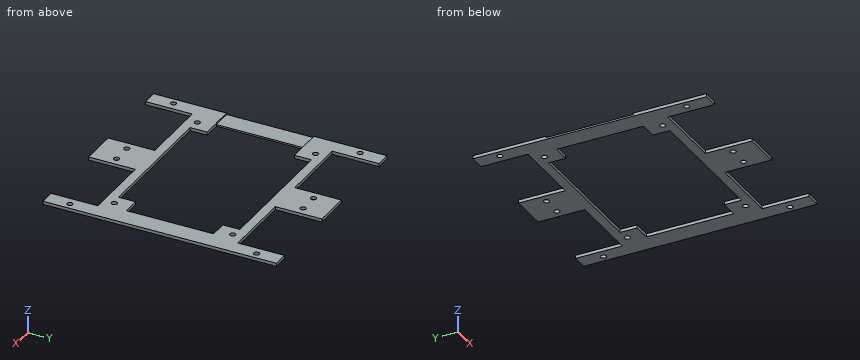
from build123d import *

# Parameters (mm, degrees)
SKETCH2_W           = 680
SKETCH2_H           = 750
BOSS_EXTRUDE1_DEPTH = 10
SKETCH3_W           = 230
SKETCH3_H           = 150
CUT_EXTRUDE1_DEPTH  = 507.285492583
SKETCH4_R           = 9
CUT_EXTRUDE4_DEPTH  = 507.285492583
SKETCH6_W           = 440
SKETCH6_H           = 280
SKETCH6_H_2         = 55
SKETCH6_W_2         = 56.5
CUT_EXTRUDE6_DEPTH  = 507.285492583
SKETCH7_W           = 63.5
SKETCH7_H           = 280.49751631
CUT_EXTRUDE7_DEPTH  = 4.6


with BuildPart() as part:
    # Sketch2 → Boss-Extrude1 (new body)
    with BuildSketch(Plane.XY):
        Rectangle(SKETCH2_W, SKETCH2_H)
    extrude(amount=BOSS_EXTRUDE1_DEPTH)

    # Sketch3 → Cut-Extrude1 (cut, through all)
    with BuildSketch(Plane.XY.offset(10)):
        with Locations((-175, 300)):
            Rectangle(SKETCH3_W, SKETCH3_H)
        with Locations((175, 300)):
            Rectangle(SKETCH3_W, SKETCH3_H)
        with Locations((175, -300)):
            Rectangle(SKETCH3_W, SKETCH3_H)
        with Locations((-175, -300)):
            Rectangle(SKETCH3_W, SKETCH3_H)
    extrude(amount=-CUT_EXTRUDE1_DEPTH, mode=Mode.SUBTRACT)

    # Sketch4 → Cut-Extrude4 (cut, through all)
    with BuildSketch(Plane.XY.offset(10)):
        with Locations((-318, 300)):
            Circle(SKETCH4_R)
        with Locations((-32, 300)):
            Circle(SKETCH4_R)
        with Locations((-255, 190)):
            Circle(SKETCH4_R)
        with Locations(Location((318, 300, 0), (0, 0, 180))):
            Circle(SKETCH4_R)
        with Locations(Location((255, 190, 0), (0, 0, 180))):
            Circle(SKETCH4_R)
        with Locations(Location((32, 300, 0), (0, 0, 180))):
            Circle(SKETCH4_R)
        with Locations((318, -300)):
            Circle(SKETCH4_R)
        with Locations((255, -190)):
            Circle(SKETCH4_R)
        with Locations((32, -300)):
            Circle(SKETCH4_R)
        with Locations(Location((-255, -190, 0), (0, 0, 180))):
            Circle(SKETCH4_R)
        with Locations(Location((-32, -300, 0), (0, 0, 180))):
            Circle(SKETCH4_R)
        with Locations(Location((-318, -300, 0), (0, 0, 180))):
            Circle(SKETCH4_R)
    extrude(amount=-CUT_EXTRUDE4_DEPTH, mode=Mode.SUBTRACT)

    # Sketch6 → Cut-Extrude6 (cut, through all)
    with BuildSketch(Plane.XY.offset(10)):
        Rectangle(SKETCH6_W, SKETCH6_H)
        with Locations((0, 167.5)):
            Rectangle(SKETCH6_W, SKETCH6_H_2)
        with Locations((0, -167.5)):
            Rectangle(SKETCH6_W, SKETCH6_H_2)
        with Locations((248.25, 0)):
            Rectangle(SKETCH6_W_2, SKETCH6_H)
        with Locations((-248.25, 0)):
            Rectangle(SKETCH6_W_2, SKETCH6_H)
    extrude(amount=-CUT_EXTRUDE6_DEPTH, mode=Mode.SUBTRACT)

    # Sketch7 → Cut-Extrude7 (cut)
    with BuildSketch(Plane.XY.offset(10)):
        with Locations((-308.25, -0.248758155)):
            Rectangle(SKETCH7_W, SKETCH7_H)
    extrude(amount=-CUT_EXTRUDE7_DEPTH, mode=Mode.SUBTRACT)


solid = part.part
Input: part model. Units: mm. Frame: model coordinates. Give positions to 0.01 mm unless a question says otherwise; leave off trailing zeros. Loops run counter-clockwise (first coordinate to the right, second up) from the corner with the lowest first, then second, coordinate; pieces in that order, holes last. Notation, with made-up numbers: M 42,-34.5 L 82,-34.5 A18 cw 82,-2.5 Z; hole C 24,-35 d7. An arc over 180 degrees is marked long. Use one line per item in the form item = value.
1. Section query D-D, the plane y = 300. Return the cut outline in (x, z), and give its area (3 significant figures).
Numbers:
outline = M -340,0 L -327,0 L -327,10 L -340,10 Z; M -309,0 L -290,0 L -290,10 L -309,10 Z; M -60,0 L -41,0 L -41,10 L -60,10 Z; M -23,0 L 23,0 L 23,10 L -23,10 Z; M 41,0 L 60,0 L 60,10 L 41,10 Z; M 290,0 L 309,0 L 309,10 L 290,10 Z; M 327,0 L 340,0 L 340,10 L 327,10 Z
area = 1,480 mm²
2. Section query B-B, the plane y = -110. Return the cut outline in (x, z).
Numbers:
outline = M -340,0 L -276.5,0 L -276.5,5.4 L -340,5.4 Z; M 276.5,0 L 340,0 L 340,10 L 276.5,10 Z
3. First-contact query: pin 1 (3 mm diameter, centred on x = 233.5, z = 1.5, fed in from -Y); pin 2 (1 mm diameter, centred on y = 69, z = 7, fed in from -X). Flat tips, straight axial feed; report the tip coordinate or a pass-through.
Numbers:
pin_1 = -225
pin_2 = 276.5
4. Section query A-A, the plane x = 170. Return the cut outline in (y, z), and give its area (3 significant figures).
Numbers:
outline = M -225,0 L -195,0 L -195,10 L -225,10 Z; M 195,0 L 225,0 L 225,10 L 195,10 Z
area = 600 mm²
5. Line query: L1, parallel to Y at x = -318, z = 6.75; L2, parallel to Y at x = 32, z = 7.5; L3, parallel to X at y = -14.5, z = 2. Output: solid intervals per line, ascending.
Numbers:
L1 = -375 to -309, -291 to -140.5, 140 to 291, 309 to 375
L2 = -375 to -309, -291 to -195, 195 to 291, 309 to 375
L3 = -340 to -276.5, 276.5 to 340
6. Section query C-C, the plane x = 318. Return the cut outline in (y, z), and give its area (3 significant figures).
Numbers:
outline = M -375,0 L -309,0 L -309,10 L -375,10 Z; M -291,0 L 291,0 L 291,10 L -291,10 Z; M 309,0 L 375,0 L 375,10 L 309,10 Z
area = 7,140 mm²
